Here's how the part is built. I have some questions about the finished solid (model axes, mm). A direction names the side the tool comes from. Round coordinates to 2 decimals unless told otherwise and drop trailing zeros. Loops run counter-clockwise (first coordinate to the right, second up) from the corner with the lowest first, then second, coordinate; pieces in that order, holes last. Notation, with made-up numbers: M -25.75,64.25 L -6.75,64.25 A18 ccw -6.75,89.25 Z; hole C -15.75,62 d2. An arc over 180 degrees is marked long. Use a Markdown table: item, result.
from build123d import *

# Parameters (mm, degrees)
F0_R     = 13
F0_R_2   = 11
F0_W     = 59
F0_H     = 2
F1_DEPTH = 9
F0_R_3   = 6
F2_DEPTH = 2
F3_W     = 26.42
F3_H     = 3.66
F4_DEPTH = 32.91456


with BuildPart() as f1:
    # F0 (on Top) → F1 (new body)
    with BuildSketch(Plane.XY):
        Polygon((13, -13.208), (13, 0), (13, 13.208), (-46, 13.208), (-46, -13.208), align=None)
        Circle(F0_R, mode=Mode.SUBTRACT)
        Circle(F0_R)
        Circle(F0_R_2, mode=Mode.SUBTRACT)
        with Locations((-16.5, 14.208)):
            Rectangle(F0_W, F0_H)
        with Locations((-16.5, -14.208)):
            Rectangle(F0_W, F0_H)
    extrude(amount=F1_DEPTH)

    # F0 (on Top) → F2 (join)
    with BuildSketch(Plane.XY):
        Circle(F0_R_2)
        Circle(F0_R_3, mode=Mode.SUBTRACT)
    extrude(amount=F2_DEPTH)

    # F3 (on face) → F4 (cut)
    with BuildSketch(Plane(origin=(-46, 0, 0), x_dir=(0, -1, 0), z_dir=(-1, 0, 0))):
        with Locations((0, 4.5)):
            Rectangle(F3_W, F3_H)
    extrude(amount=-F4_DEPTH, mode=Mode.SUBTRACT)


solid = f1.part
1. Which directions (+Z, -Z, +X, -X, +Y, -Y) give clear straight access to the entire face, cutting with the end or side of a thin tool? Please do faces 1 (the face through (-46, 0, 2)), 2 (the face through (-30, 13.21, 4)), 3 (the face through (-2.38, -10.74, 5.45)).
Answer sheet:
| item | result |
|---|---|
| face 1 | +Z, -Z, -X, +Y, -Y |
| face 2 | -X |
| face 3 | +Z |
2. For pin 1 Ø17.5 at (x, y) = (-1.5, -1.5) entering from +Z; pin 2 Ø7 at (x, y) = (0, 0) entering from +Z, each with a flat end and sliding along its axis, tell me the tip position at first contact or that it passes through.
Answer sheet:
| item | result |
|---|---|
| pin 1 | z = 2 |
| pin 2 | through |
3. Imagine slicing it at B-B, the plane z = 5.25. Write out the boundary of the cut face in (x, y), then the cut area to 3 significant figures.
Answer sheet:
| item | result |
|---|---|
| outline | M -46,-15.21 L 13,-15.21 L 13,15.21 L -46,15.21 L -46,13.21 L -13.09,13.21 L -13.09,-13.21 L -46,-13.21 Z; hole C 0,0 d22 |
| area | 545 mm2 |
4. We'd pull the mould along Y, two halves only. Please class faces 4 (the face through (-17, -15.208, 4)), 5 (the face through (-23, 0, 9)), 6 (the face through (5, -5, 2)): +Y half, -Y half, draft (parallel to the pull), parting line (faces both ways), or undercut.
Answer sheet:
| item | result |
|---|---|
| face 4 | -Y half |
| face 5 | draft |
| face 6 | undercut |
5. I need wall thicknesses on probe 1 along Z at (x, y) = (-21.5, 4); probe 2 along Y at (x, z) = (0, 1.65); probe 3 along X at (y, z) = (-13, 6.25). Which ranges of each line are inside material? Lowest first, please. Write a range as from..to.
Answer sheet:
| item | result |
|---|---|
| probe 1 | 0..2.67, 6.33..9 |
| probe 2 | -15.21..-6, 6..15.21 |
| probe 3 | -13.09..13 |
6. Imagine slicing it at C-C, the plane y = 0. Write out the boundary of the cut face in (x, z).
Answer sheet:
| item | result |
|---|---|
| outline | M -46,0 L -6,0 L -6,2 L -11,2 L -11,9 L -46,9 L -46,6.33 L -13.09,6.33 L -13.09,2.67 L -46,2.67 Z; M 6,0 L 13,0 L 13,9 L 11,9 L 11,2 L 6,2 Z |
7. Imagine slicing it at D-D, the plane z = 8. Write out the boundary of the cut face in (x, y), then the cut area to 3 significant figures.
Answer sheet:
| item | result |
|---|---|
| outline | M -46,-15.21 L 13,-15.21 L 13,15.21 L -46,15.21 Z; hole C 0,0 d22 |
| area | 1,410 mm2 |
8. Imagine slicing it at A-A, the plane x = 0. Write out the boundary of the cut face in (y, z).
Answer sheet:
| item | result |
|---|---|
| outline | M -15.21,0 L -6,0 L -6,2 L -11,2 L -11,9 L -15.21,9 Z; M 6,0 L 15.21,0 L 15.21,9 L 11,9 L 11,2 L 6,2 Z |
